```python
from build123d import *

# Parameters (mm, degrees)
F0_W     = 2.7374038473
F0_H     = 4.5464726281
F0_W_2   = 2.3603244432
F0_H_2   = 20.3094583448
F1_DEPTH = 3


with BuildPart() as f1:
    # F0 (on Front) → F1 (new body)
    with BuildSketch(Plane.XZ):
        with BuildLine():
            Line((-13.9879264009, 8.4983842463), (-10.7078288449, 8.4983842463))
            ThreePointArc((-10.7078288449, 8.4983842463), (-12.3096819162, -5.9457433928), (0, -13.6704108706))
            Line((0, -13.6704108706), (29.832560569, -13.6704108706))
            ThreePointArc((29.832560569, -13.6704108706), (41.0439649972, -7.8220549805), (42.6626390029, 4.7190275219))
            ThreePointArc((42.6626390029, 4.7190275219), (52.7277631814, 0.6811115523), (57.2114773095, -9.193492122))
            Line((57.2114773095, -9.193492122), (57.2114773095, 27.5829305145))
            ThreePointArc((57.2114773095, 27.5829305145), (52.7277631814, 17.7083268402), (42.6626390029, 13.6704108706))
            Line((42.6626390029, 13.6704108706), (29.832560569, 13.6704108706))
            Line((29.832560569, 13.6704108706), (0, 13.6704108706))
            Line((0, 13.6704108706), (-14.4307379611, 13.6704108706))
            Line((-14.4307379611, 13.6704108706), (-14.8297163701, 14.5122008398))
            Line((-14.8297163701, 14.5122008398), (-15.268201828, 14.5122008398))
            ThreePointArc((-15.268201828, 14.5122008398), (-15.9753086092, 14.219307621), (-16.268201828, 13.5122008398))
            Line((-16.268201828, 13.5122008398), (-16.268201828, 9.0994058373))
            ThreePointArc((-16.268201828, 9.0994058373), (-15.9753086092, 8.3922990562), (-15.268201828, 8.0994058373))
            Line((-15.268201828, 8.0994058373), (-14.8297163701, 8.0994058373))
            Line((-14.8297163701, 8.0994058373), (-13.9879264009, 8.4983842463))
        make_face()
        with Locations((-10.5523099191, -3.12910098)):
            Rectangle(F0_W, F0_H, mode=Mode.SUBTRACT)
        Polygon((5.7225638777, -7.545285929), (5.7225638777, -9.6566872671), (-5.59899235, -9.6566872671), (-5.59899235, 10.6527710777), (5.7225638777, 10.6527710777), (5.7225638777, 8.5547049059), (-3.2386679067, 8.5547049059), (-3.2386679067, 2.0115832855), (5.180267113, 2.0115832855), (5.180267113, -0.0731477199), (-3.2386679067, -0.0731477199), (-3.2386679067, -7.545285929), align=None, mode=Mode.SUBTRACT)
        with Locations((-10.5523099191, 3.0826488801)):
            Rectangle(F0_W, F0_H, mode=Mode.SUBTRACT)
        with BuildLine():
            Line((21.1113458408, -9.6566872671), (19.2088621088, -9.6566872671))
            Line((19.2088621088, -9.6566872671), (12.3190261635, 8.3457872998))
            Line((12.3190261635, 8.3457872998), (12.2078997772, 8.3457872998))
            add(Edge.make_bspline(
                [(12.2078997772, 8.3457872998), (12.403482217, 6.207715629), (12.403482217, 3.2606438666)],
                knots=[0, 0, 0, 1, 1, 1], degree=2))
            Line((12.403482217, 3.2606438666), (12.403482217, -9.6566872671))
            Line((12.403482217, -9.6566872671), (10.2209599917, -9.6566872671))
            Line((10.2209599917, -9.6566872671), (10.2209599917, 10.6527710777))
            Line((10.2209599917, 10.6527710777), (13.7770043506, 10.6527710777))
            Line((13.7770043506, 10.6527710777), (20.2089995848, -6.1006429082))
            Line((20.2089995848, -6.1006429082), (20.320125971, -6.1006429082))
            Line((20.320125971, -6.1006429082), (26.8054618705, 10.6527710777))
            Line((26.8054618705, 10.6527710777), (30.3348358968, 10.6527710777))
            Line((30.3348358968, 10.6527710777), (30.3348358968, -9.6566872671))
            Line((30.3348358968, -9.6566872671), (27.9745114535, -9.6566872671))
            Line((27.9745114535, -9.6566872671), (27.9745114535, 3.4295559736))
            add(Edge.make_bspline(
                [(27.9745114535, 3.4295559736), (27.9745114535, 5.6787540306), (28.1700938933, 8.3191169671)],
                knots=[0, 0, 0, 1, 1, 1], degree=2))
            Line((28.1700938933, 8.3191169671), (28.0589675071, 8.3191169671))
            Line((28.0589675071, 8.3191169671), (21.1113458408, -9.6566872671))
        make_face(mode=Mode.SUBTRACT)
        with Locations((37.0846525955, 0.4980419053)):
            Rectangle(F0_W_2, F0_H_2, mode=Mode.SUBTRACT)
    extrude(amount=F1_DEPTH)


solid = f1.part
```
Build history of the part. All positions in model axes, mm. A direction names the side the tool comes from. Round coordinates to 2 decimals unless told otherwise and drop trailing zeros. Loops run counter-clockwise (first coordinate to the right, second up) from the corner with the lowest first, then second, coordinate; pieces in that order, holes last.
Item 1: Saw through at D-D (x = -10). List the corners of the cut face in (y, z).
Item 2: Drill centre lines: line 1 along Z through (x, y) = (2, -0.2); line 2 along Z through (x, y) = (29.5, -0.2); line 3 along Z through (x, y) = (-1.5, -2.4). Where is each one in solid material? Low to high.
Item 3: Two-plate mould, pull along X, no slides. Class faces 1 (the face through (29, -1, 10.653)), 2 (the face through (15, -1, -13.67)), 3 (the face through (57.211, -1, 9)): released by +X, released by -X, zero draft, split by the parting line, or undercut.
Item 4: Saw through at A-A (x = 3.5). List the corners of the cut face in (y, z).
Item 5: Which spindle directions (+Z, -Z, +X, -X, +Y, -Y) get a long thin tool onto all of the face, cutting with end or side? Do faces 4 (the face through (0, -1, -9.657)), 5 (the face through (15, -1, 13.67)). Say none if no direction does.
Item 6: Saw through at B-B (x = 22.5). List the corners of the cut face in (y, z).
Item 7: Pin check, flat tips, straight feed: P1, Ø0.5, axis at x = -15, y = -2, coming from the +Z side; P2, Ø1.2, axis at x = 29.5, y = -1.5, coming from the +Z side; P3, Ø0.9, axis at y = -1, z = -2.5, coming from the -X side. Stop position of each tip, or through.
Item 8: Saw through at C-C (y = -1.7). State how many separate pieces and enclosed holes the cut face has, then the cut area to 3 significant figures.
Worked answers:
1. outline: (-3, -9.32) - (0, -9.32) - (0, -5.4) - (-3, -5.4) - close; (-3, -0.86) - (0, -0.86) - (0, 0.81) - (-3, 0.81) - close; (-3, 5.36) - (0, 5.36) - (0, 13.67) - (-3, 13.67) - close
2. line 1: z = -13.67 to -9.66, -7.55 to -0.07, 2.01 to 8.55, 10.65 to 13.67
2. line 2: z = -13.67 to -9.66, 10.65 to 13.67
2. line 3: z = -13.59 to -9.66, -7.55 to -0.07, 2.01 to 8.55, 10.65 to 13.67
3. face 1: undercut
3. face 2: zero draft
3. face 3: released by +X
4. outline: (-3, -13.67) - (0, -13.67) - (0, -9.66) - (-3, -9.66) - close; (-3, -7.55) - (0, -7.55) - (0, -0.07) - (-3, -0.07) - close; (-3, 2.01) - (0, 2.01) - (0, 8.55) - (-3, 8.55) - close; (-3, 10.65) - (0, 10.65) - (0, 13.67) - (-3, 13.67) - close
5. face 4: +Y, -Y
5. face 5: +Z, +Y, -Y
6. outline: (-3, -13.67) - (0, -13.67) - (0, -6.06) - (-3, -6.06) - close; (-3, -0.47) - (0, -0.47) - (0, 13.67) - (-3, 13.67) - close
7. P1: stops at z = 14.51
7. P2: stops at z = 13.67
7. P3: stops at x = -13.52
8. separate pieces: 1
8. enclosed holes: 5
8. area: 1,350 mm2
